Source: CAD feature listing. Evaluate the final solid. Frame: model axes, mm. Face numbers are marked on the shaded views. Give positions to 0.01 mm unless a question says otherwise; leave off trailing zeros. Loops run counter-clockwise (first coordinate to the right, second up) from the corner with the lowest first, then second, coordinate; pieces in that order, holes last.
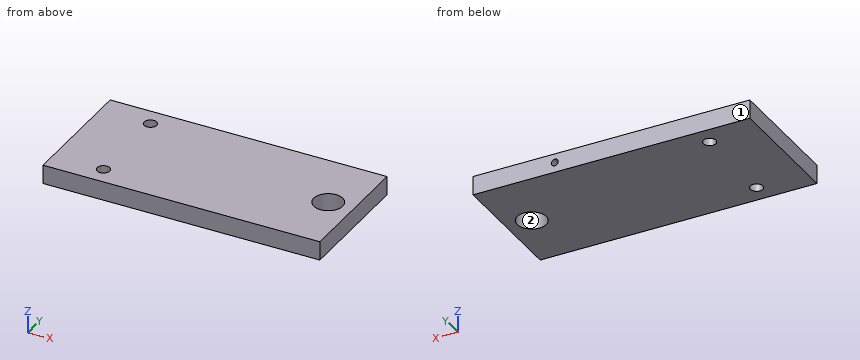
from build123d import *

# Parameters (mm, degrees)
SKETCH1_W                   = 139.7
SKETCH1_H                   = 63.5
BOSS_EXTRUDE1_DEPTH         = 9.525
F_5_8_18_TAPPED_HOLE1_D     = 14.68374
F_1_4_0_25_DIAMETER_HOLE1_D = 6.35
F_8_32_TAPPED_HOLE1_D       = 3.4544
F_8_32_TAPPED_HOLE1_DEPTH   = 12.7
F_8_32_TAPPED_HOLE1_TIP     = 1.037806461


with BuildPart() as part:
    # Sketch1 → Boss-Extrude1 (new body)
    with BuildSketch(Plane.XY):
        with Locations((69.85, 31.75)):
            Rectangle(SKETCH1_W, SKETCH1_H)
    extrude(amount=BOSS_EXTRUDE1_DEPTH)

    # 5/8-18 Tapped Hole1 (through all)
    with Locations(Plane.XY.offset(9.525)):
        with Locations((127, 31.75)):
            Hole(F_5_8_18_TAPPED_HOLE1_D / 2)

    # 1/4 (0.25) Diameter Hole1 (through all)
    with Locations(Plane(origin=(25.4, 53.975, 9.525), x_dir=(1, 0, 0), z_dir=(0, 0, 1))):
        with Locations((0, 0), (0, -44.45)):
            Hole(F_1_4_0_25_DIAMETER_HOLE1_D / 2)

    # #8-32 Tapped Hole1
    with Locations(Plane(origin=(98.425, 63.5, 5.08), x_dir=(0, 0, 1), z_dir=(0, 1, 0))):
        with Locations((0, 0)):
            Hole(F_8_32_TAPPED_HOLE1_D / 2, depth=F_8_32_TAPPED_HOLE1_DEPTH)
            with Locations((0, 0, -(F_8_32_TAPPED_HOLE1_DEPTH + F_8_32_TAPPED_HOLE1_TIP / 2))):  # 118° drill point
                Cone(0, F_8_32_TAPPED_HOLE1_D / 2, F_8_32_TAPPED_HOLE1_TIP, mode=Mode.SUBTRACT)


solid = part.part
1) Cut plane B-B (x = 127). Return loops of the section in (y, z) (3 decimals), and give its area (3 significant figures).
Checks:
outline: (0, 0) - (24.408, 0) - (24.408, 9.525) - (0, 9.525) - close; (39.092, 0) - (63.5, 0) - (63.5, 9.525) - (39.092, 9.525) - close
area: 465 mm2
2) Ray query, probe 1 along Y at (x, z) = (25.4, 4.5); probe 2 along Y at (x, z) = (127, 3.5); probe 3 along X at (y, z) = (59.5, 5.08). Return the intervals inside material, ascending.
Checks:
probe 1: y = 0 to 6.35, 12.7 to 50.8, 57.15 to 63.5
probe 2: y = 0 to 24.41, 39.09 to 63.5
probe 3: x = 0 to 96.7, 100.15 to 139.7
3) Cut plane A-A (y = 31.75). Return loops of the section in (x, z) (3 decimals), and give its area (3 significant figures).
Checks:
outline: (0, 0) - (119.658, 0) - (119.658, 9.525) - (0, 9.525) - close; (134.342, 0) - (139.7, 0) - (139.7, 9.525) - (134.342, 9.525) - close
area: 1,190 mm2
4) Contact query for a flat-ended pin moving along its axis: P1, Ø2, axis at x = 98.425, z = 5.08, coming from the +Y side. Output: stop coordinate, or through.
Checks:
P1: stops at y = 50.36
5) Pull-direction query (X, two-part tool) for the marked faces 1 and 2; classes: released by +X, released by -X, zero draft, split by the parting line, or undercut.
Checks:
face 1: zero draft
face 2: undercut
